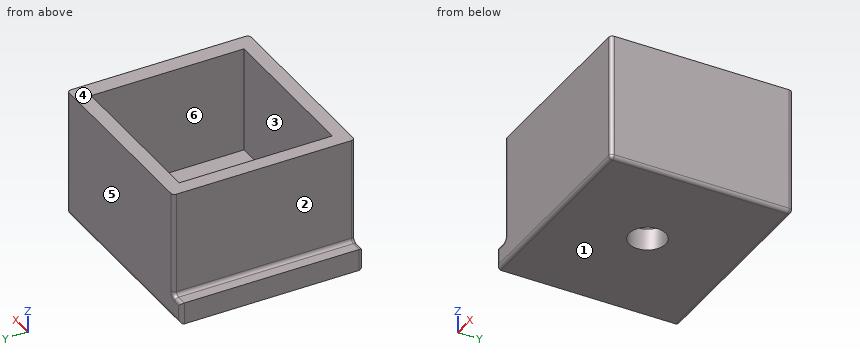
```python
from build123d import *

# Parameters (mm, degrees)
ESBO_O1_W                = 56
ESBO_O1_H                = 50
ESBO_O1_R                = 5
RESSALTO_EXTRUS_O1_DEPTH = 6
ESBO_O2_W                = 52.1
ESBO_O2_H                = 50
ESBO_O2_W_2              = 43.5
ESBO_O2_H_2              = 42
RESSALTO_EXTRUS_O2_DEPTH = 29
FILETE1_R                = 1


with BuildPart() as part:
    # Esboço1 → Ressalto-extrusão1 (new body)
    with BuildSketch(Plane.XY):
        with Locations((4.281632844, -11.096885813)):
            Rectangle(ESBO_O1_W, ESBO_O1_H)
        with Locations((5.491632844, -11.096885813)):
            Circle(ESBO_O1_R, mode=Mode.SUBTRACT)
    extrude(amount=RESSALTO_EXTRUS_O1_DEPTH)

    # Esboço2 → Ressalto-extrusão2 (add)
    with BuildSketch(Plane.XY.offset(6)):
        with Locations((6.231632844, -11.096885813)):
            Rectangle(ESBO_O2_W, ESBO_O2_H)
        with Locations((5.931632844, -11.096885813)):
            Rectangle(ESBO_O2_W_2, ESBO_O2_H_2, mode=Mode.SUBTRACT)
    extrude(amount=RESSALTO_EXTRUS_O2_DEPTH)

    # Filete1
    filete1_edges = [part.edges().sort_by_distance(p)[0] for p in [
        (-21.768367156, 13.903114187, 6),
        (-19.818367156, -11.096885813, 6),
        (-19.818367156, 13.903114187, 20.5),
        (-19.818367156, -36.096885813, 20.5),
        (4.281632844, 13.903114187, 0),
        (32.281632844, -11.096885813, 0),
        (4.281632844, -36.096885813, 0),
        (-23.718367156, 13.903114187, 3),
        (32.281632844, 13.903114187, 17.5),
        (32.281632844, -36.096885813, 17.5),
        (-23.718367156, -36.096885813, 3),
        (-21.768367156, -36.096885813, 6),
    ]]
    fillet(filete1_edges, radius=FILETE1_R)


solid = part.part
```
CAD build for the part. Positions are in the model's coordinates, mm. Face numbers are marked on the shaded views. A direction names the side the tool comes from. Round coordinates to 2 decimals unless told otherwise and drop trailing zeros. Order: outer loops, then holes, each group sorted by start corner. A loop starts at its lowest first (then second) coordinate and runs counter-clockwise, first axis right, second up. Notation, with made-up numbers: (82.25, 27.5) - (97.25, 27.5) arc R26 cw to (97.25, 44.5) - close; hole circle Ø9 at (4.25, 53). An arc over 180 degrees is marked (long way). Answer in a Markdown table with one row per item. Add a question column.
(1) 3-axis set-ups, long thin cutter, end or side, ignore diameter. For the marked faces 1, 2 and 3: which of +Z, -Z, +X, -X, +Y, -Y reach the whole face in a straight line?
(2) Probe L1, parallel to Y at x = 9, z = 6.5; L2, parallel to X at y = -9.5, z = 24; L3, parallel to Z at x = 19.5, y = 5. List the from-to ranges inside material, lowest first. Write a range as [from, to].
(3) Band-saw the part on D-D on x = -5. List the corners of the cut face in (y, z), and give its area (3 significant figures).
(4) Drop flat-ended pins along their axis: pin 1 Ø14 at (y, z) = (-7.5, 24) entering from -X; pin 2 Ø21 at (x, y) = (15, -3.5) entering from +Z. Give the stop position or say it passes through.
(5) Mould opens along Y. For the marked faces 4, 5 and 6 say: +Y half, -Y half, draft (parallel to the pull), parting line (faces both ways), or undercut.
(6) Band-saw the part on A-A on z = 11. List the corners of the cut face in (x, y), and give its area (3 significant figures).
(7) Band-saw the part on C-C on y = -5. List the corners of the cut face in (x, z), and give its area (3 significant figures).
(8) Band-saw the part on B-B on x = 4. List the corners of the cut face in (y, z).
Data:
| question | item | result |
|---|---|---|
| 1 | face 1 | -Z, +X, -X, +Y, -Y |
| 1 | face 2 | +Z, -X, +Y, -Y |
| 1 | face 3 | +Z |
| 2 | L1 | y = [-36.1, -32.1], [9.9, 13.9] |
| 2 | L2 | x = [-19.82, -15.82], [27.68, 32.28] |
| 2 | L3 | z = [0, 6] |
| 3 | outline | (-36.1, 1) arc R1 ccw to (-35.1, 0) - (12.9, 0) arc R1 ccw to (13.9, 1) - (13.9, 35) - (9.9, 35) - (9.9, 6) - (-32.1, 6) - (-32.1, 35) - (-36.1, 35) - close |
| 3 | area | 532 mm^2 |
| 4 | pin 1 | stops at x = -19.82 |
| 4 | pin 2 | stops at z = 6 |
| 5 | face 4 | draft |
| 5 | face 5 | +Y half |
| 5 | face 6 | undercut |
| 6 | outline | (-19.82, -35.1) arc R1 ccw to (-18.82, -36.1) - (31.28, -36.1) arc R1 ccw to (32.28, -35.1) - (32.28, 12.9) arc R1 ccw to (31.28, 13.9) - (-18.82, 13.9) arc R1 ccw to (-19.82, 12.9) - close; hole (-15.82, -32.1) - (27.68, -32.1) - (27.68, 9.9) - (-15.82, 9.9) - close |
| 6 | area | 777 mm^2 |
| 7 | outline | (-23.72, 0) - (31.28, 0) arc R1 ccw to (32.28, 1) - (32.28, 35) - (27.68, 35) - (27.68, 6) - (-15.82, 6) - (-15.82, 35) - (-19.82, 35) - (-19.82, 7) arc R1 cw to (-20.82, 6) - (-23.72, 6) - close |
| 7 | area | 585 mm^2 |
| 8 | outline | (-36.1, 1) arc R1 ccw to (-35.1, 0) - (-15.87, 0) - (-15.87, 6) - (-32.1, 6) - (-32.1, 35) - (-36.1, 35) - close; (-6.32, 0) - (12.9, 0) arc R1 ccw to (13.9, 1) - (13.9, 35) - (9.9, 35) - (9.9, 6) - (-6.32, 6) - close |
